```python
from build123d import *

# Parameters (mm, degrees)
F0_W          = 14.224
F0_H          = 3.556
F1_DEPTH      = 25.4
F1_DEPTH_BACK = 31.75
F2_W          = 5.08
F2_H          = 5.08
F3_DEPTH      = 3.556
F3_DEPTH_BACK = 3.556
F4_W          = 1.905
F4_H          = 4.572
F5_DEPTH      = 3.81
F5_DEPTH_BACK = 3.81


with BuildPart() as f1:
    # F0 (on Front) → F1 (new body, two sides)
    with BuildSketch(Plane.XZ) as f1_sk:
        with Locations((-0.0590678749, 0.0447268487)):
            Rectangle(F0_W, F0_H)
    extrude(amount=F1_DEPTH)
    extrude(f1_sk.sketch, amount=-F1_DEPTH_BACK)

    # F2 (on Right) → F3 (join, two sides)
    with BuildSketch(Plane.YZ) as f3_sk:
        with Locations((-22.8598152912, 4.2202161699)):
            Rectangle(F2_W, F2_H)
    extrude(amount=F3_DEPTH)
    extrude(f3_sk.sketch, amount=-F3_DEPTH_BACK)

    # F4 (on Right) → F5 (cut, two sides)
    with BuildSketch(Plane.YZ) as f5_sk:
        with Locations((-22.1804035014, 4.6287587003)):
            Rectangle(F4_W, F4_H)
    extrude(amount=-F5_DEPTH, mode=Mode.SUBTRACT)
    extrude(f5_sk.sketch, amount=F5_DEPTH_BACK, mode=Mode.SUBTRACT)


solid = f1.part
```
Build history of the part. All positions in model axes, mm. A direction names the side the tool comes from. Coordinates: 2 decimals unless noted, no trailing zeros. Order: outer loops, then holes, each group sorted by start corner. A loop starts at its lowest first (then second) coordinate and runs counter-clockwise, first axis right, second up. Notation, with made-up numbers: M 57.5,-23.5 L 110.5,-23.5 A23 ccw 110.5,-15.5 Z; hole C 18.25,-36 d6. An arc over 180 degrees is marked long. One line per question, with ' | ' between items. Start each with the question number.
1. Mould opens along Y. For faces 1 (the face through (0, 31.75, 0)), 2 (the face through (3.556, -23.5, 4.3)), 3 (the face through (0, -21.228, 5)) say: +Y half, -Y half, draft (parallel to the pull), parting line (faces both ways), or undercut.
2. Cut at C-C (y = -15). Write the cut outline in (x, z).
3. Tool access for faces 4 (the face through (7.053, 3, 0)), 5 (the face through (-3.556, -23.5, 4.3)), 6 (the face through (0, -20.32, 4)), 7 (the face through (0, -23.133, 5)), 8 (the face through (0, -24, 6.76)): list every direction of +Z, -Z, +X, -X, +Y, -Y with a clear straight run to the whole face (end or side of a thin tool).
4. Flat gauge pins, fed straight in: P1, Ø4.5, axis at x = -2.5, y = -6, coming from the +Z side; P2, Ø1.5, axis at x = -1, z = 5.5, coming from the +Y side; P3, Ø2.5, axis at y = -23, z = 5, coming from the -X side. Where does each tip first touch, or does it go through?
5. Cut at D-D (x = 6). Write the cut outline in (y, z), plus the area to 3 significant figures.
6. Cut at A-A (z = 4). Write the cut outline in (x, y).
7. Wall check: line 1 along Y through (x, z) = (1.5, 3); line 2 along Z through (x, y) = (-0.75, 18.5); line 3 along Y through (x, z) = (-1, 2). Give the ranges that are in metal, low to high. Write a range as [from, to].
The answers:
1) face 1: +Y half | face 2: draft | face 3: undercut
2) outline: M -7.17,-1.73 L 7.05,-1.73 L 7.05,1.82 L -7.17,1.82 Z
3) face 4: +Z, -Z, +X, +Y, -Y | face 5: +Z, -X, +Y, -Y | face 6: +Z, +X, -X, +Y | face 7: +Z, +X, -X | face 8: +Z, +X, -X, +Y, -Y
4) P1: stops at z = 1.82 | P2: stops at y = -20.32 | P3: stops at x = -3.56
5) outline: M -25.4,-1.73 L 31.75,-1.73 L 31.75,1.82 L -25.4,1.82 Z | area: 203 mm2
6) outline: M -3.56,-25.4 L 3.56,-25.4 L 3.56,-23.13 L -3.56,-23.13 Z; M -3.56,-21.23 L 3.56,-21.23 L 3.56,-20.32 L -3.56,-20.32 Z
7) line 1: y = [-25.4, -23.13], [-21.23, -20.32] | line 2: z = [-1.73, 1.82] | line 3: y = [-25.4, -20.32]
